Read the model definition and answer for the solid it produces. Units are mm, in the model's axes. A direction names the side the tool comes from. Round coordinates to 2 decimals unless told otherwise and drop trailing zeros. Order: outer loops, then holes, each group sorted by start corner. A loop starts at its lowest first (then second) coordinate and runs counter-clockwise, first axis right, second up. Notation, with made-up numbers: (-27, -35.75) - (29, -35.75) arc R37 cw to (29, 0.25) - close; hole circle Ø3 at (65.25, 34). An arc over 180 degrees is marked (long way). Answer as a JSON object with one key per item and string values. Group by question number.
Q1. The mould has two halves that part along Z. Classify faces 3 (the flat face through (10, 2.75, 0)), 4 (the cylindrical face through (1.39, 14.4, -9.43)), 5 (the cylindrical face through (1.356, 7.926, -6.461)): pulls with the +Z half, pulls with the -Z half, needs draft (parallel to the pull), parting line crosses it, or undercut.
Q2. A cutting plane is placed at D-D on x = 2.5. Determine the outline of the cut face in (y, z) (3 decimals), and give its area (3 significant figures).
Q3. Consider line 1 (Y direction, x = 2, z = -6) (3 decimals); line 2 (Z direction, x = 11, y = 2) (3 decimals). Determine where each line is inside the solid, lowest interval first.
Q4. A tool of negligible diameter and unlimited length cuts with its end or side. For faces 1 (the flat face through (4, 2, 10)), 2 (the flat face through (2.75, 10, 0)), from which of +Z, -Z, +X, -X, +Y, -Y can it reach the whole face along a straight path? Write none if from no direction.
Q5. A cutting plane is placed at C-C on z = -6. Determine the outline of the cut face in (x, y) (3 decimals).
Q6. A cutting plane is placed at A-A on x = 10. Determine the outline of the cut face in (y, z) (3 decimals), and give its area (3 significant figures).
Q7. Given pin 1 Ø4 at (x, z) = (10, 6) entering from -Y; pin 2 Ø6 at (y, z) = (7.5, -0.5) entering from +X; pin 3 Ø8 at (x, z) = (7.5, 0.5) entering from +Y, each flat-ended and moving along its own axis, determine where each tip first touches the part or whether it passes through.
```python
from build123d import *

# Parameters (mm, degrees)
SKETCH3_W           = 15
SKETCH3_H           = 20
SKETCH3_R           = 2.125
BOSS_EXTRUDE3_DEPTH = 2.75
SKETCH5_W           = 20
SKETCH5_H           = 15
SKETCH5_R           = 2.125
BOSS_EXTRUDE5_DEPTH = 2.75
FILLET4_R           = 2


with BuildPart() as part:
    # Sketch3 → Boss-Extrude3 (new body)
    with BuildSketch(Plane(origin=(0, 0, 0), x_dir=(1, 0, 0), z_dir=(0, 1, 0))):
        with Locations((7.5, 0)):
            Rectangle(SKETCH3_W, SKETCH3_H)
        with Locations(Location((10, 6, 0), (0, 0, 270))):
            Circle(SKETCH3_R, mode=Mode.SUBTRACT)
        with Locations(Location((10, -6, 0), (0, 0, 90))):
            Circle(SKETCH3_R, mode=Mode.SUBTRACT)
    extrude(amount=BOSS_EXTRUDE3_DEPTH)

    # Sketch5 → Boss-Extrude5 (add)
    with BuildSketch(Plane.ZY):
        with Locations((0, 7.5)):
            Rectangle(SKETCH5_W, SKETCH5_H)
        with Locations((-6, 10)):
            Circle(SKETCH5_R, mode=Mode.SUBTRACT)
        with Locations(Location((6, 10, 0), (0, 0, 180))):
            Circle(SKETCH5_R, mode=Mode.SUBTRACT)
    extrude(amount=-BOSS_EXTRUDE5_DEPTH)

    # Fillet4
    fillet4_edges = [part.edges().sort_by_distance(p)[0] for p in [
        (1.375, 15, 10),
        (1.375, 15, -10),
        (2.75, 2.75, 0),
        (15, 1.375, 10),
        (15, 1.375, -10),
    ]]
    fillet(fillet4_edges, radius=FILLET4_R)


solid = part.part
```
Result set:
{
 "1": {"face 3": "needs draft", "face 4": "pulls with the -Z half", "face 5": "undercut"},
 "2": {"outline": "(0, -10) - (13, -10) arc R2 ccw to (15, -8) - (15, 8) arc R2 ccw to (13, 10) - (0, 10) - close; hole circle Ø4.25 at (10, -6); hole circle Ø4.25 at (10, 6)", "area": "270 mm²"},
 "3": {"line 1": "y = 0 to 7.875, 12.125 to 15", "line 2": "z = -10 to -7.875, -4.125 to 4.125, 7.875 to 10"},
 "4": {"face 1": "+Z, +X, -X, +Y, -Y", "face 2": "+Z, -Z, +X, +Y"},
 "5": {"outline": "(0, 0) - (7.875, 0) - (7.875, 2.75) - (4.75, 2.75) arc R2 cw to (2.75, 4.75) - (2.75, 7.875) - (0, 7.875) - close; (0, 12.125) - (2.75, 12.125) - (2.75, 15) - (0, 15) - close; (12.125, 0) - (15, 0) - (15, 2.75) - (12.125, 2.75) - close"},
 "6": {"outline": "(0, -10) - (2.75, -10) - (2.75, -8.125) - (0, -8.125) - close; (0, -3.875) - (2.75, -3.875) - (2.75, 3.875) - (0, 3.875) - close; (0, 8.125) - (2.75, 8.125) - (2.75, 10) - (0, 10) - close", "area": "31.6 mm²"},
 "7": {"pin 1": "passes through", "pin 2": "stops at x = 2.77", "pin 3": "stops at y = 3.19"}
}
